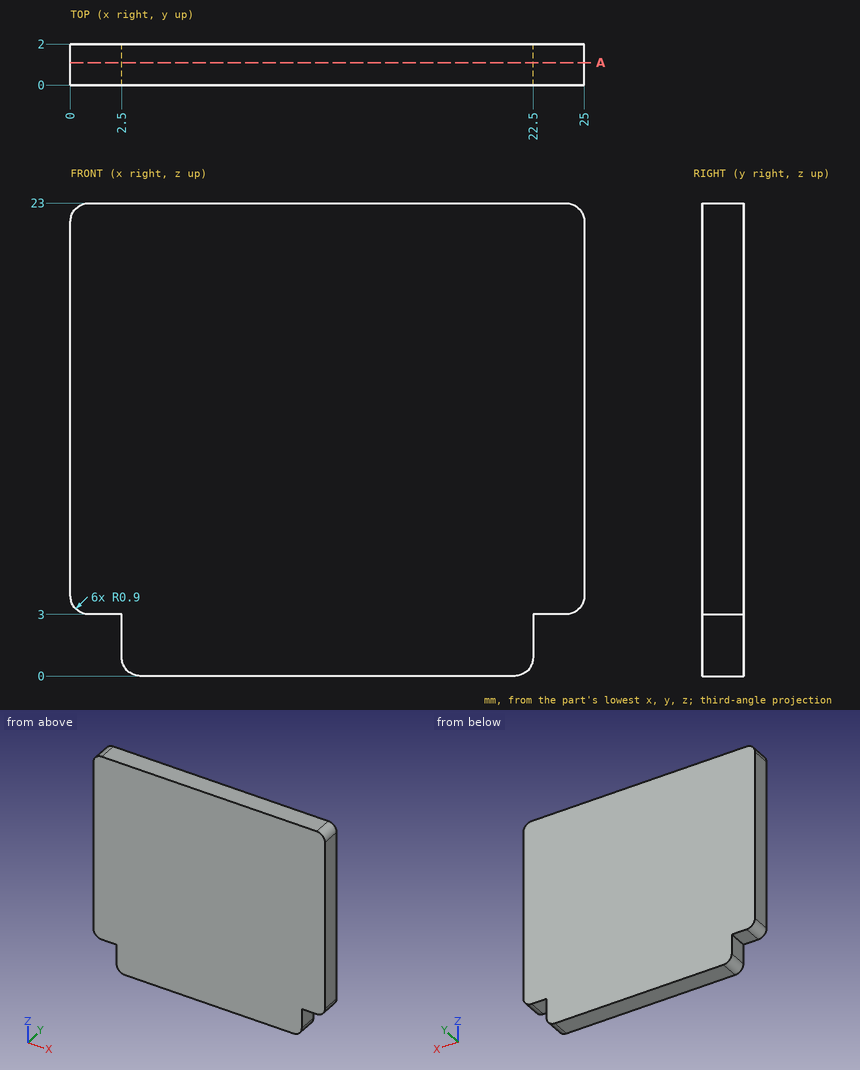
Drawing for the job (mm, zero at the part's lowest x, y, z). Round coordinates to 2 decimals unless told otherwise and drop trailing zeros. Loops run counter-clockwise (first coordinate to the right, second up) from the corner with the lowest first, then second, coordinate; pieces in that order, holes last.
1. Drop flat-ended pins along their axis: P1, Ø1, axis at x = 7, z = 16.5, coming from the -Y side; P2, Ø0.5, axis at x = 1.5, y = 1, coming from the -Z side; P3, Ø0.6, axis at y = 1, z = 2.5, coming from the -X side. Give the stop position or say it passes through.
Check values:
P1: stops at y = 0
P2: stops at z = 3
P3: stops at x = 2.5
2. Band-saw the part on A-A, the plane y = 1.1. List the corners of the cut face in (x, z).
Check values:
outline: (0, 3.9) arc R0.9 ccw to (0.9, 3) - (2.5, 3) - (2.5, 0.9) arc R0.9 ccw to (3.4, 0) - (21.6, 0) arc R0.9 ccw to (22.5, 0.9) - (22.5, 3) - (24.1, 3) arc R0.9 ccw to (25, 3.9) - (25, 22.1) arc R0.9 ccw to (24.1, 23) - (0.9, 23) arc R0.9 ccw to (0, 22.1) - close
3. Wall check: probe 1 along Z at (x, y) = (2, 1.35); probe 2 along Z at (x, y) = (3, 0.75); probe 3 along X at (y, z) = (1.9, 3.75). Give the ranges that are in metal, low to high.
Check values:
probe 1: z = 3 to 23
probe 2: z = 0.09 to 23
probe 3: x = 0.01 to 24.99
